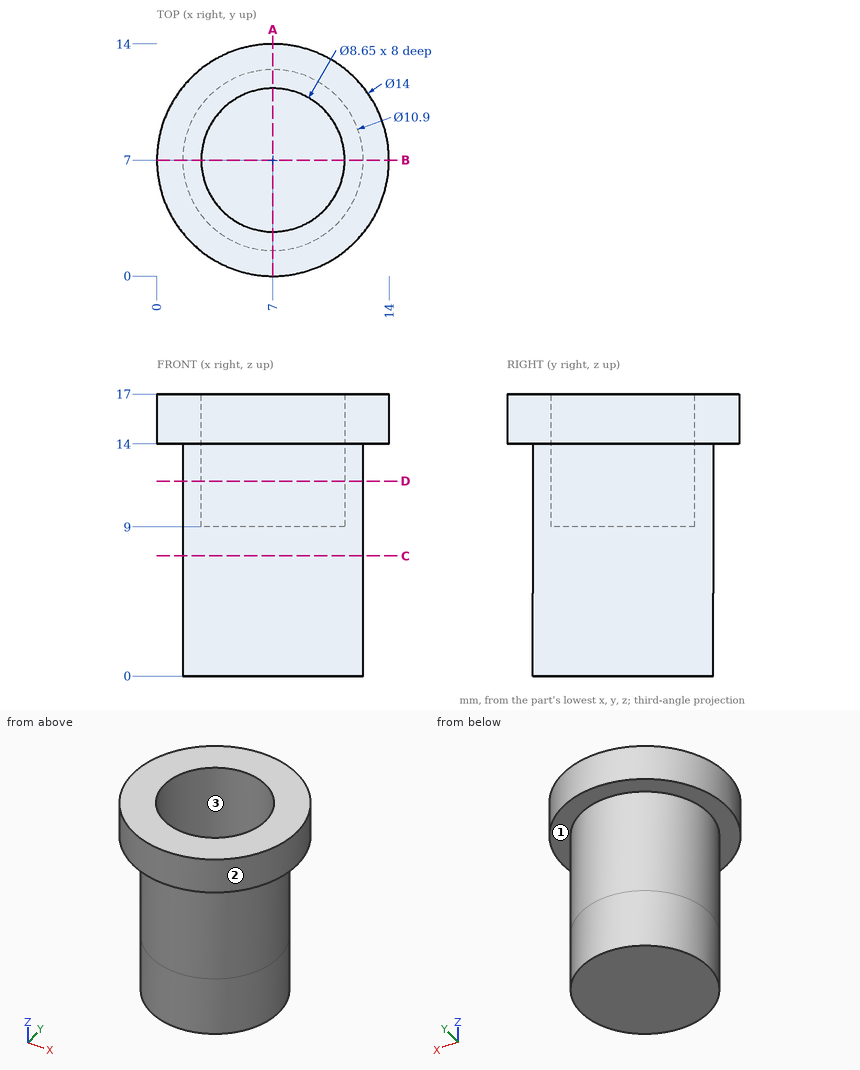
For this review, use the dimensioned drawing (mm, ordinates from the lowest corner) and the shaded views. Coordinates: 2 decimals unless noted, no trailing zeros. Write each loop counter-clockwise with the first axis right and the second up, starting at its lowest first coordinate (ties: lowest second). Pieces come first, ordered by that corner, then holes. Notation, with made-up numbers: (-14.5, 44.25) - (29.5, 44.25) arc R18 ccw to (29.5, 52.25) - close; hole circle Ø8 at (14.25, -27.75). An arc over 180 degrees is marked (long way). Answer in a Markdown table with one row per item. Add a question column.
Q1. Consider section A-A on x = 7. Give the boundary of the cut face in (y, z) (3 decimals), then the cut area to 3 significant figures.
Q2. Consider section D-D on z = 11.75. Give the boundary of the cut face in (x, y) (3 decimals), then the cut area to 3 significant figures.
Q3. Clearance check with flat-ended pins moving along their axes: pin 1 (8 mm diameter, centred on x = 5, z = 5, fed in from +Y); pin 2 (3 mm diameter, centred on y = 2.5, z = 14.5, fed in from -X); pin 3 (1.5 mm diameter, centred on y = 7.5, z = 6.5, fed in from +X); pin 4 (1 mm diameter, centred on x = 1.5, y = 1.5, fed in from +Z). State where each tip first meets the part, or that it passes through.
Q4. Draft analysis for pull direction X (two halves, no side actions). For the marked faces 1, 2 and 3, state which applies: +X half, -X half, draft (parallel to the pull), parting line (faces both ways), or undercut.
Q5. Consider section C-C on z = 7.25. Give the boundary of the cut face in (x, y).
Q6. To check wall thickness, follow line 1 along Y through (x, z) = (7, 12.75) (3 decimals); line 2 along Y through (x, z) = (7, 14.5) (3 decimals); line 3 along Z through (x, y) = (13, 5.75). State the ranges of each line that lie inside material, in increasing order. Write a range as from..to.
Answers below:
| question | item | result |
|---|---|---|
| 1 | outline | (0, 14) - (1.55, 14) - (1.55, 0) - (12.45, 0) - (12.45, 14) - (14, 14) - (14, 17) - (11.325, 17) - (11.325, 9) - (2.675, 9) - (2.675, 17) - (0, 17) - close |
| 1 | area | 125 mm² |
| 2 | outline | circle Ø10.9 at (7, 7); hole circle Ø8.65 at (7, 7) |
| 2 | area | 34.5 mm² |
| 3 | pin 1 | y = 12.45 |
| 3 | pin 2 | x = 0.68 |
| 3 | pin 3 | x = 12.45 |
| 3 | pin 4 | through |
| 4 | face 1 | draft |
| 4 | face 2 | parting line |
| 4 | face 3 | undercut |
| 5 | outline | circle Ø10.9 at (7, 7) |
| 6 | line 1 | 1.55..2.675, 11.325..12.45 |
| 6 | line 2 | 0..2.675, 11.325..14 |
| 6 | line 3 | 14..17 |
